```python
from build123d import *

# Parameters (mm, degrees)
F0_W     = 60
F0_H     = 30
F1_DEPTH = 30
F2_R     = 11
F3_DEPTH = 20
F4_W     = 9
F4_H     = 9
F5_DEPTH = 31
F6_R     = 6
F7_DEPTH = 26
F8_SIZE2 = 10
F8_SIZE  = 30
F9_R     = 3


with BuildPart() as f1:
    # F0 (on Front) → F1 (new body)
    with BuildSketch(Plane.XZ):
        Rectangle(F0_W, F0_H)
    extrude(amount=F1_DEPTH)

    # F2 (on face) → F3 (cut)
    with BuildSketch(Plane.XZ.offset(30)):
        with Locations((-15, 0)):
            Circle(F2_R)
    extrude(amount=-F3_DEPTH, mode=Mode.SUBTRACT)

    # F4 (on face) → F5 (cut)
    with BuildSketch(Plane.YZ.offset(30)):
        with Locations((-15, -7.5)):
            Rectangle(F4_W, F4_H)
    extrude(amount=-F5_DEPTH, mode=Mode.SUBTRACT)

    # F6 (on face) → F7 (cut)
    with BuildSketch(Plane.XY.offset(15)):
        with Locations((-15, -15)):
            Circle(F6_R)
    extrude(amount=-F7_DEPTH, mode=Mode.SUBTRACT)

    # F8
    f8_edges = [f1.edges().sort_by_distance(p)[0] for p in [
        (30, -15, 15),
    ]]
    f8_side = f1.faces().sort_by_distance((1.005666, -15, 15))[0]
    chamfer(f8_edges, length=F8_SIZE, length2=F8_SIZE2, reference=f8_side)

    # F9
    f9_edges = [f1.edges().sort_by_distance(p)[0] for p in [
        (-30, -15, 15),
        (-15, 0, 15),
        (0, -15, 15),
        (30, -15, 5),
        (-15, -30, 15),
        (15, -30, 10),
        (15, 0, 10),
        (30, -30, -5),
        (30, 0, -5),
        (-30, 0, 0),
        (-30, -30, 0),
    ]]
    fillet(f9_edges, radius=F9_R)


with BuildPart() as f10_1:
    # F10: instance of F1
    add(f1.part.mirror(Plane.XZ.offset(30)))


solid = f10_1.part
```
Read the model definition and answer for the solid it produces. Units are mm, in the model's axes. A direction names the side the tool comes from. Give positions to 0.01 mm unless a question says otherwise; leave off trailing zeros. Loops run counter-clockwise (first coordinate to the right, second up) from the corner with the lowest first, then second, coordinate; pieces in that order, holes last.
Item 1: The part is cut by section A-A (y = -38). Write down the section's boundary in (x, z).
Item 2: Find the intervals of material crossed by line 1 along Y through (x, z) = (-15, 6); line 2 along X through (y, z) = (-43.5, 5.5); line 3 along Y through (x, z) = (-23.5, -5.5), in increasing order.
Item 3: The mould has two halves that part along Y. Classify faces 1 (the flat face through (15, -40.5, -8)), 2 (the cylindrical face through (14.112, -59.145, 9.345)), 3 (the cylindrical face through (14.127, -30.902, 9.389)): released by +Y, released by -Y, zero draft, split by the parting line, or undercut.
Item 4: Each of these flat-tipped pins is pushed along its axis until it touches: pin 1 Ø4 at (x, z) = (-23.5, 0) entering from +Y; pin 2 Ø2.5 at (y, z) = (-44.5, -9.5) entering from +X; pin 3 Ø9.5 at (x, y) = (-15, -45) entering from +Z. Where does it stop, or does it pass through?
Item 5: The part is cut by section D-D (y = -55). Write down the section's boundary in (x, z), and give its area (3 significant figures).
Item 6: For faces 4 (the flat face through (0, -60, -1)), 5 (the flat face through (15, -49.5, -8)), 6 (the cylindrical face through (-16.432, -37.638, 10.906)), determine the directions among +Z, -Z, +X, -X, +Y, -Y from which every point of the face is accessible in a straight line to the end or side of a thin tool.
Item 7: The part is cut by section C-C (x = -10.5). Write down the section's boundary in (y, z), and give its area (3 significant figures).
Item 8: The part is cut by section B-B (z = 0). Write down the section's boundary in (x, y), and give its area (3 significant figures).
Taken from the geometry:
1. outline: (-30, -15) - (30, -15) - (30, 2.84) arc R3 ccw to (27.95, 5.68) - (0.46, 14.85) arc R3 ccw to (-0.49, 15) - (-27, 15) arc R3 ccw to (-30, 12) - close; hole circle Ø22 at (-15, 0)
2. line 1: y = -60 to -51
2. line 2: x = -30 to -24.53, -5.47 to 28.38
2. line 3: y = -60 to -50
3. face 1: undercut
3. face 2: released by -Y
3. face 3: released by +Y
4. pin 1: stops at y = -50
4. pin 2: stops at x = -1
4. pin 3: stops at z = -11
5. outline: (-30, -15) - (30, -15) - (30, 2.84) arc R3 ccw to (27.95, 5.68) - (0.46, 14.85) arc R3 ccw to (-0.49, 15) - (-27, 15) arc R3 ccw to (-30, 12) - close
5. area: 1,650 mm2
6. face 4: +Z, -Z, +X, -X, -Y
6. face 5: +X
6. face 6: +Y
7. outline: (-60, -15) - (-30, -15) - (-30, -10.04) - (-41.03, -10.04) - (-41.03, -11) - (-48.97, -11) - (-48.97, -10.04) - (-50, -10.04) - (-50, 10.04) - (-48.97, 10.04) - (-48.97, 15) - (-57, 15) arc R3 ccw to (-60, 12) - close; (-41.03, 10.04) - (-30, 10.04) - (-30, 12) arc R3 ccw to (-33, 15) - (-41.03, 15) - close
7. area: 448 mm2
8. outline: (-30, -57) arc R3 ccw to (-27, -60) - (27, -60) arc R3 ccw to (30, -57) - (30, -33) arc R3 ccw to (27, -30) - (-4, -30) - (-4, -50) - (-11.68, -50) arc R6 cw to (-18.32, -50) - (-26, -50) - (-26, -30) - (-27, -30) arc R3 ccw to (-30, -33) - close
8. area: 1,350 mm2
